Input: part model. Units: mm. Frame: model coordinates. Face numbers are marked on the shaded views. A direction names the side the tool comes from. Give positions to 0.01 mm unless a question says otherwise; leave off trailing zeros. Loops run counter-clockwise (first coordinate to the right, second up) from the corner with the lowest first, then second, coordinate; pieces in that order, holes last. Notation, with made-up numbers: (-1, 38) -> (39, 38) arc R15 cw to (39, 63) -> close; hole circle Ø1 at (-20, 38). An arc over 180 degrees is marked (long way). Answer as a JSON object with one key per item and string values. Group by question number.
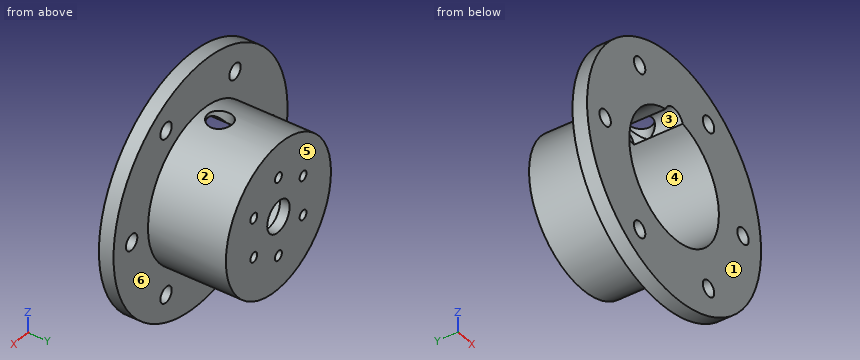
```python
from build123d import *

# Parameters (mm, degrees)
SKETCH2_R          = 1
SKETCH2_R_2        = 1.65
CUT_EXTRUDE1_DEPTH = 41.449042016
CIRPATTERN1_COUNT  = 6
SKETCH3_R          = 2.5
CUT_EXTRUDE2_DEPTH = 38.220626002
CUT_EXTRUDE3_START = -10
CUT_EXTRUDE3_DEPTH = 10


with BuildPart() as part:
    # Sketch1 → Revolve1 (revolve)
    with BuildSketch(Plane.XY, mode=Mode.PRIVATE) as revolve1_sk:
        Polygon((3.25, 8.5), (3.25, 10.5), (15.25, 10.5), (15.25, -5.5), (25.25, -5.5), (25.25, -8.5), (13, -8.5), (13, 8.5), align=None)
    revolve(revolve1_sk.sketch.rotate(Axis((0, -8.78125, 0), (0, 1, 0)), 90), axis=Axis((0, -8.78125, 0), (0, 1, 0)))

    # Sketch2 → Cut-Extrude1 (cut, through all)
    with BuildSketch(Plane(origin=(0, 10.5, 0), x_dir=(1, 0, 0), z_dir=(0, 1, 0))):
        with Locations(Location((0, 8.25, 0), (0, 0, 270))):
            Circle(SKETCH2_R)
        with Locations(Location((20, 0, 0), (0, 0, 270))):
            Circle(SKETCH2_R_2)
    cut_extrude1 = extrude(amount=-CUT_EXTRUDE1_DEPTH, mode=Mode.SUBTRACT)

    # CirPattern1: Cut-Extrude1 ×6 about axis
    cirpattern1_axis = Axis((0, 0, 0), (0, 1, 0))
    for i in range(1, CIRPATTERN1_COUNT):
        add(cut_extrude1.rotate(cirpattern1_axis, i * 360 / CIRPATTERN1_COUNT), mode=Mode.SUBTRACT)

    # Sketch3 → Cut-Extrude2 (cut, through all)
    with BuildSketch(Plane.XY):
        with Locations(Location((0, -1.5, 0), (0, 0, 180))):
            Circle(SKETCH3_R)
    extrude(amount=CUT_EXTRUDE2_DEPTH, mode=Mode.SUBTRACT)

    # Sketch4 → Cut-Extrude3 (cut)
    with BuildSketch(Plane.XZ.offset(8.5).offset(CUT_EXTRUDE3_START)):
        with BuildLine():
            ThreePointArc((2.5, 12.757350822), (0, 13), (-2.5, 12.757350822))
            ThreePointArc((-2.5, 12.757350822), (0, 14.5), (2.5, 12.757350822))
        make_face()
    extrude(amount=CUT_EXTRUDE3_DEPTH, mode=Mode.SUBTRACT)


solid = part.part
```
Q1. Set-up query: the marked faces 4, 5 and 6. Return all of +Z, -Z, +X, -X, +Y, -Y with unobstructed straight access to the full face (end or side cutting, diameter ignored); none if empty.
Q2. Section D-D on x = -10. Return the cut outline in (y, z).
Q3. Pull-direction query (X, two-part tool) for the marked faces 1, 2 and 3; classes: +X half, -X half, draft (parallel to the pull), parting line (faces both ways), or undercut.
Q4. Ray query, probe 1 along X at (y, z) = (-7.2, 0); probe 2 along Y at (x, z) = (22.5, 8.5); probe 3 along X at (y, z) = (8.75, 2.5). Return the intervals inside material, ascending.
Q5. Section B-B on z = 0. Return the cut outline in (x, y).
Q6. Pin query (flat end, axial travel): pin 1 Ø10 at (x, y) = (-5.5, 7) entering from -Z; pin 2 Ø1.8 at (x, z) = (0, 8.25) entering from +Y; pin 3 Ø2.5 at (x, z) = (0, -8.25) entering from -Y; pin 4 Ø4 at (y, z) = (5.5, -2.5) entering from +X. Return the tip coordinate at first contact, or that it passes through.
Q7. Section C-C on z = 8.25. Return the cut outline in (x, y), then the cut area to 3 significant figures.
Q8. Section A-A on x = 0. State how many separate pieces and enclosed holes the cut face has, then the cut area to 3 significant figures.
Numbers:
{
 "1": {"face 4": "-Y", "face 5": "+Z, -Z, +X, -X, +Y", "face 6": "+Y"},
 "2": {"outline": "(-8.5, -23.19) -> (-5.5, -23.19) -> (-5.5, -18.97) -> (-8.5, -18.97) -> close; (-8.5, -15.67) -> (-5.5, -15.67) -> (-5.5, -11.51) -> (10.5, -11.51) -> (10.5, 11.51) -> (-5.5, 11.51) -> (-5.5, 15.67) -> (-8.5, 15.67) -> (-8.5, 8.31) -> (8.5, 8.31) -> (8.5, -8.31) -> (-8.5, -8.31) -> close; (-8.5, 18.97) -> (-5.5, 18.97) -> (-5.5, 23.19) -> (-8.5, 23.19) -> close"},
 "3": {"face 1": "draft", "face 2": "parting line", "face 3": "undercut"},
 "4": {"probe 1": "x = -25.25 to -21.65, -18.35 to -13, 13 to 18.35, 21.65 to 25.25", "probe 2": "y = -8.5 to -5.5", "probe 3": "x = -15.04 to -2.08, 2.08 to 15.04"},
 "5": {"outline": "(-25.25, -8.5) -> (-21.65, -8.5) -> (-21.65, -5.5) -> (-25.25, -5.5) -> close; (-18.35, -8.5) -> (-13, -8.5) -> (-13, 8.5) -> (-3.25, 8.5) -> (-3.25, 10.5) -> (-15.25, 10.5) -> (-15.25, -5.5) -> (-18.35, -5.5) -> close; (3.25, 8.5) -> (13, 8.5) -> (13, -8.5) -> (18.35, -8.5) -> (18.35, -5.5) -> (15.25, -5.5) -> (15.25, 10.5) -> (3.25, 10.5) -> close; (21.65, -8.5) -> (25.25, -8.5) -> (25.25, -5.5) -> (21.65, -5.5) -> close"},
 "6": {"pin 1": "stops at z = -15.24", "pin 2": "passes through", "pin 3": "stops at y = 8.5", "pin 4": "stops at x = 15.24"},
 "7": {"outline": "(-23.86, -8.5) -> (-10.05, -8.5) -> (-10.05, 8.5) -> (-1, 8.5) -> (-1, 10.5) -> (-12.83, 10.5) -> (-12.83, -5.5) -> (-23.86, -5.5) -> close; (1, 8.5) -> (10.05, 8.5) -> (10.05, -8.5) -> (23.86, -8.5) -> (23.86, -5.5) -> (12.83, -5.5) -> (12.83, 10.5) -> (1, 10.5) -> close", "area": "208 mm²"},
 "8": {"separate pieces": "5", "enclosed holes": "0", "area": "158 mm²"}
}
